```python
from build123d import *

# Parameters (mm, degrees)
F0_R     = 44.5
F0_R_2   = 5.5
F0_R_3   = 11.1
F1_DEPTH = 7
F2_R     = 5.5526911935
F3_R     = 5.5
F4_DEPTH = 3.5


# Not quite as in the source:
# - a fillet or chamfer that OpenCascade refuses, or shapes differently, is made with other operations: its cross-section is extruded or revolved along the edge and cut away or added


with BuildPart() as f1:
    # F0 (on Top) → F1 (new body)
    with BuildSketch(Plane.XY):
        with Locations((1.3388e-06, 0.0960128228)):
            Circle(F0_R)
        with Locations((-19.7783853119, -19.7235588551)):
            Circle(F0_R_2, mode=Mode.SUBTRACT)
        with Locations((19.7783879895, -19.7235588551)):
            Circle(F0_R_2, mode=Mode.SUBTRACT)
        with Locations((1.3388e-06, 0.0960128228)):
            Circle(F0_R_3, mode=Mode.SUBTRACT)
        with Locations((0.0567746402, 28.095976607)):
            Circle(F0_R_2, mode=Mode.SUBTRACT)
    extrude(amount=F1_DEPTH)

    # F2
    f2_edges = [f1.edges().sort_by_distance(p)[0] for p in [
        (-44.499999, 0.096013, 7),
    ]]
    fillet(f2_edges, radius=F2_R)

    # F3 (on face) → F4 (join)
    with BuildSketch(Plane.XY.offset(7)):
        with Locations((20.2050062432, 20.8988438036)):
            Circle(F3_R)
        with Locations((28.9993370366, 0.292301098)):
            Circle(F3_R)
        with Locations((1.3388e-06, -28.9039871772)):
            Circle(F3_R)
        with Locations((-28.9925298787, -0.5621160422)):
            Circle(F3_R)
        with Locations((-20.7871988103, 20.3170985988)):
            Circle(F3_R)
    extrude(amount=F4_DEPTH)

    # F5: fillet of radius 5.5 on 5 edges, made by hand

    # F5_s1 → F5_t2 (revolve, cut)
    with BuildSketch(Plane.XZ.offset(0.5621160422)):
        with BuildLine():
            ThreePointArc((-23.4925298787, 7), (-25.5135868502, 9.5414755311), (-28.6160052617, 10.5))
            Line((-28.6160052617, 10.5), (-23.4925298787, 10.5))
            Line((-23.4925298787, 10.5), (-23.4925298787, 7))
        make_face()
    revolve(axis=Axis((-28.9925298787, -0.5621160422, 10.5), (0, 0, 1)), mode=Mode.SUBTRACT)

    # F5_s3 → F5_t4 (revolve, cut)
    with BuildSketch(Plane.XZ.offset(-20.3170985988)):
        with BuildLine():
            ThreePointArc((-15.2871988103, 7), (-17.3082557818, 9.5414755311), (-20.4106741933, 10.5))
            Line((-20.4106741933, 10.5), (-15.2871988103, 10.5))
            Line((-15.2871988103, 10.5), (-15.2871988103, 7))
        make_face()
    revolve(axis=Axis((-20.7871988103, 20.3170985988, 10.5), (0, 0, 1)), mode=Mode.SUBTRACT)

    # F5_s5 → F5_t6 (revolve, cut)
    with BuildSketch(Plane.XZ.offset(-20.8988438036)):
        with BuildLine():
            ThreePointArc((25.7050062432, 7), (23.6839492717, 9.5414755311), (20.5815308602, 10.5))
            Line((20.5815308602, 10.5), (25.7050062432, 10.5))
            Line((25.7050062432, 10.5), (25.7050062432, 7))
        make_face()
    revolve(axis=Axis((20.2050062432, 20.8988438036, 10.5), (0, 0, 1)), mode=Mode.SUBTRACT)

    # F5_s7 → F5_t8 (revolve, cut)
    with BuildSketch(Plane.XZ.offset(-0.292301098)):
        with BuildLine():
            ThreePointArc((34.4993370366, 7), (32.4782800651, 9.5414755311), (29.3758616536, 10.5))
            Line((29.3758616536, 10.5), (34.4993370366, 10.5))
            Line((34.4993370366, 10.5), (34.4993370366, 7))
        make_face()
    revolve(axis=Axis((28.9993370366, 0.292301098, 10.5), (0, 0, 1)), mode=Mode.SUBTRACT)

    # F5_s9 → F5_t10 (revolve, cut)
    with BuildSketch(Plane.XZ.offset(28.9039871772)):
        with BuildLine():
            ThreePointArc((5.5000013388, 7), (3.4789443673, 9.5414755311), (0.3765259558, 10.5))
            Line((0.3765259558, 10.5), (5.5000013388, 10.5))
            Line((5.5000013388, 10.5), (5.5000013388, 7))
        make_face()
    revolve(axis=Axis((1.3388e-06, -28.9039871772, 10.5), (0, 0, 1)), mode=Mode.SUBTRACT)


solid = f1.part
```
Here's how the part is built. I have some questions about the finished solid (model axes, mm). A direction names the side the tool comes from. Give positions to 0.01 mm unless a question says otherwise; leave off trailing zeros. Write each loop counter-clockwise with the first axis right and the second up, starting at its lowest first coordinate (ties: lowest second). Pieces come first, ordered by that corner, then holes. Notation, with made-up numbers: M -14.5,34 L 10.5,34 A17 ccw 10.5,41 Z; hole C 15,28.5 d4. An arc over 180 degrees is marked long. Put each result on its own line as item: value. Start each with the question number.
Item 1: On a 3-axis mill with a long thin cutter (end or side, diameter ignored), from which of +Z, -Z, +X, -X, +Y, -Y can I reach the whole of each face in a straight line? I mean faces 1 (the cylindrical face through (-23.832, -16.006, 3.451)), 2 (the flat face through (8, -8, 7)). Say none if no direction works.
Item 2: Will these pins go through, and if not, where does the flat tip stop? pin 1 (2 mm diameter, centred on x = 23, z = 9, fed in from +Y); pin 2 (14.5 mm diameter, centred on x = -19.78, y = -19.72, fed in from +Z); pin 3 (1 mm diameter, centred on y = -7.5, z = 6, fed in from -X); pin 4 (18 mm diameter, centred on x = 0, y = 0.1, fed in from +Z).
Item 3: If we section it at B-B, the plane x = 1.5: Count the separate pieces of the cut face and the enclosed holes in it, then the cut area to 3 significant figures.
Item 4: Thinking about a two-plate mould opening in Y: for faces 3 (the cylindrical face through (42.445, 13.463, 0.714)), 4 (the flat face through (9, -9, 0)), 5 (the cylindrical face through (19.06, -14.27, 3.45)), which applies, +Y half, -Y half, draft (parallel to the pull), parting line (faces both ways), or undercut?
Item 5: If we section it at A-A, the plane z = 3.75: Write out the boundary of the cut face in (x, y), then the cut area to 3 significant figures.
Item 6: I need wall thicknesses on L1, parallel to Y at x = 5, z = 6.5; L2, parallel to Z at x = 2, y = -39; L3, parallel to Y at x = 4.5, z = 1.75. Which ranges of each line are inside material? Lowest first, please. Write a range as from..to.
Values:
1. face 1: +Z, -Z
1. face 2: +Z
2. pin 1: y = 25.23
2. pin 2: z = 7
2. pin 3: x = -42.07
2. pin 4: through
3. separate pieces: 3
3. enclosed holes: 0
3. area: 407 mm²
4. face 3: parting line
4. face 4: draft
4. face 5: undercut
5. outline: C 0,0.1 d88; hole C -19.78,-19.72 d11; hole C 0,0.1 d22.2; hole C 0.06,28.1 d11; hole C 19.78,-19.72 d11
5. area: 5,410 mm²
6. L1: -40.85..-9.81, 10.01..25.68, 30.51..41.04
6. L2: 0..7
6. L3: -44.17..-10.05, 10.24..24.85, 31.34..44.36
